from build123d import *

# Parameters (mm, degrees)
SKETCH_1_R          = 1.5
EXTRUDE_1_DEPTH     = 3.5
SKETCH_2_W          = 8.3
SKETCH_2_H          = 1.4
SKETCH_2_W_2        = 12.3
SKETCH_2_H_2        = 5.7
CUT_EXTRUDE_1_DEPTH = 0.5
SKETCH_2_3_W        = 9.6
SKETCH_2_3_H        = 3.1
CUT_EXTRUDE_2_DEPTH = 1
CUT_EXTRUDE_3_DEPTH = 2


with BuildPart() as part:
    # Sketch 1 → Extrude 1 (new body)
    with BuildSketch(Plane(origin=(0, 0, 0), x_dir=(1, 0, 0), z_dir=(0, 1, 0))):
        with BuildLine():
            Line((-42, -25), (42, -25))
            ThreePointArc((42, -25), (44.121320344, -24.121320344), (45, -22))
            Line((45, -22), (45, 22))
            ThreePointArc((45, 22), (44.121320344, 24.121320344), (42, 25))
            Line((42, 25), (-42, 25))
            ThreePointArc((-42, 25), (-44.121320344, 24.121320344), (-45, 22))
            Line((-45, 22), (-45, -22))
            ThreePointArc((-45, -22), (-44.121320344, -24.121320344), (-42, -25))
        make_face()
        with Locations(Location((-39, 19, 0), (0, 0, 270))):
            Circle(SKETCH_1_R, mode=Mode.SUBTRACT)
        with Locations(Location((39, 19, 0), (0, 0, 270))):
            Circle(SKETCH_1_R, mode=Mode.SUBTRACT)
        with Locations(Location((-39, -19, 0), (0, 0, 270))):
            Circle(SKETCH_1_R, mode=Mode.SUBTRACT)
        with Locations(Location((39, -19, 0), (0, 0, 270))):
            Circle(SKETCH_1_R, mode=Mode.SUBTRACT)
    extrude(amount=EXTRUDE_1_DEPTH)

    # Sketch 2 → Cut-Extrude 1 (cut)
    with BuildSketch(Plane(origin=(0, 3.5, 0), x_dir=(1, 0, 0), z_dir=(0, 1, 0))):
        with Locations((-25, 21.2)):
            Rectangle(SKETCH_2_W, SKETCH_2_H)
        with Locations((25, 22.15)):
            Rectangle(SKETCH_2_W_2, SKETCH_2_H_2)
    extrude(amount=-CUT_EXTRUDE_1_DEPTH, mode=Mode.SUBTRACT)

    # Sketch 2_3 → Cut-Extrude 2 (cut)
    with BuildSketch(Plane(origin=(0, 3.5, 0), x_dir=(1, 0, 0), z_dir=(0, 1, 0))):
        with Locations((-25, 23.45)):
            Rectangle(SKETCH_2_3_W, SKETCH_2_3_H)
    extrude(amount=-CUT_EXTRUDE_2_DEPTH, mode=Mode.SUBTRACT)

    # Sketch 3 → Cut-Extrude 3 (cut)
    with BuildSketch(Plane.XZ):
        Polygon((-37.4988893, 21.6), (-40.5011107, 21.6), (-42.0022214, 19), (-40.5011107, 16.4), (-37.4988893, 16.4), (-35.9977786, 19), align=None)
        Polygon((-37.4988893, -16.4), (-40.5011107, -16.4), (-42.0022214, -19), (-40.5011107, -21.6), (-37.4988893, -21.6), (-35.9977786, -19), align=None)
        Polygon((40.5011107, -16.4), (37.4988893, -16.4), (35.9977786, -19), (37.4988893, -21.6), (40.5011107, -21.6), (42.0022214, -19), align=None)
        Polygon((37.4988893, 21.6), (35.9977786, 19), (37.4988893, 16.4), (40.5011107, 16.4), (42.0022214, 19), (40.5011107, 21.6), align=None)
    extrude(amount=-CUT_EXTRUDE_3_DEPTH, mode=Mode.SUBTRACT)


solid = part.part
Check sheet for the modelled part. Datum: model origin and axes. Units: mm. A direction names the side the tool comes from. Round coordinates to 2 decimals unless told otherwise and drop trailing zeros. Order: outer loops, then holes, each group sorted by start corner. A loop starts at its lowest first (then second) coordinate and runs counter-clockwise, first axis right, second up.
(1) Cross-section at B-B, the plane y = 0.85. State how many separate pieces and enclosed holes the cut face has, and give its area (3 significant figures).
(2) Draft check along Z on faces 1 (the cylindrical face through (44.14, 1.73, -24.1)), 2 (the flat face through (-1, 0, 0)), 3 (the cylindrical face through (38.1, 2.7, -20.2)). Enter one of: pulls with the +Z half, pulls with the -Z half, needs draft (parallel to the pull), parting line crosses it, or undercut.
(3) Cross-section at A-A, the plane x = -39. Enter the section's corners in (y, z), and give its area (3 significant figures).
(4) Access from +Z, -Z, +X, -X, +Y, -Y to the whole of each face (thin tool, end or side, straight path). Record for faces 4 (the cylindrical face through (-44.1, 1.73, -24.14)), 5 (the flat face through (41.24, 0.99, 17.68)).
(5) Scan lines: probe 1 along X at (y, z) = (2.7, 19); probe 2 along Z at (x, y) = (40, 1); probe 3 along Z at (x, y) = (-39, 2.4). Record each from-to range of solid material in increasing order.
(6) Cross-section at C-C, the plane x = 28. Enter the section's corners in (y, z), and give its area (3 significant figures).
(7) Go/stop test with flat-tipped pins: P1, Ø1.8, axis at x = 39, z = 19, coming from the +Y side; P2, Ø1.1, axis at x = -24.5, y = 3, coming from the -Z side; P3, Ø1.1, axis at y = 3, z = -23, coming from the -X side; P4, Ø0.6, axis at y = 3.5, z = -23, coming from the -X side. Record where each tip stops, or that it passes through.
Check sheet entries:
1. separate pieces: 1
1. enclosed holes: 4
1. area: 4,400 mm2
2. face 1: pulls with the -Z half
2. face 2: needs draft
2. face 3: undercut
3. outline: (0, -25) - (3.5, -25) - (3.5, -20.5) - (2, -20.5) - (2, -21.6) - (0, -21.6) - close; (0, -16.4) - (2, -16.4) - (2, -17.5) - (3.5, -17.5) - (3.5, 17.5) - (2, 17.5) - (2, 16.4) - (0, 16.4) - close; (0, 21.6) - (2, 21.6) - (2, 20.5) - (3.5, 20.5) - (3.5, 25) - (0, 25) - close
3. area: 145 mm2
4. face 4: -Z, -X, +Y, -Y
4. face 5: -Y
5. probe 1: x = -45 to -40.5, -37.5 to 37.5, 40.5 to 45
5. probe 2: z = -25 to -21.6, -16.4 to 16.4, 21.6 to 25
5. probe 3: z = -25 to -20.5, -17.5 to 17.5, 20.5 to 25
6. outline: (0, -25) - (3, -25) - (3, -19.3) - (3.5, -19.3) - (3.5, 25) - (0, 25) - close
6. area: 172 mm2
7. P1: passes through
7. P2: stops at z = -25
7. P3: stops at x = -44.97
7. P4: stops at x = -44.92
